Design review of the part built by this model. Coordinates are the model's own, in mm. Face numbers are marked on the shaded views. A direction names the side the tool comes from. Give positions to 0.01 mm unless a question says otherwise; leave off trailing zeros. Order: outer loops, then holes, each group sorted by start corner. A loop starts at its lowest first (then second) coordinate and runs counter-clockwise, first axis right, second up. Notation, with made-up numbers: (13.5, 58) -> (20.5, 58) arc R27 ccw to (20.5, 97) -> close; hole circle Ø7 at (39, 6.5). An arc over 180 degrees is marked (long way). Return JSON: item names as keys, results as strings.
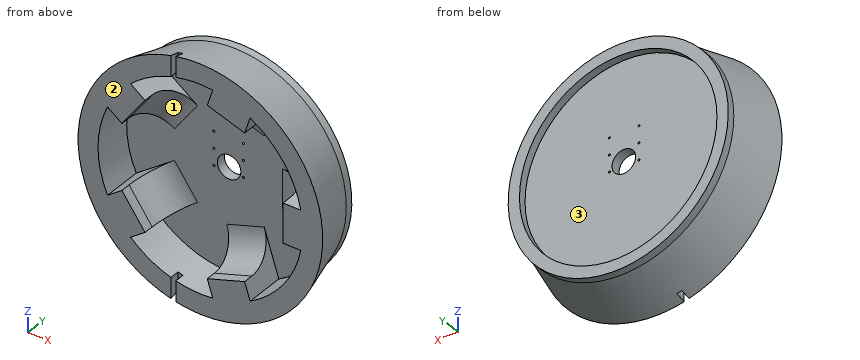
```python
from build123d import *

# Parameters (mm, degrees)
SKETCH10_R              = 1.025
CUT_EXTRUDE2_DEPTH      = 10
SKETCH11_R              = 112
SKETCH11_R_2            = 100.5
BOSS_EXTRUDE1_DEPTH     = 7.75
BOSS_EXTRUDE2_DEPTH     = 20
CIRPATTERN1_COUNT       = 5
CUT_EXTRUDE3_DEPTH      = 285.75526773
CUT_EXTRUDE3_DEPTH_BACK = 285.75526773
SKETCH14_W              = 5
SKETCH14_H              = 10


with BuildPart() as part:
    # Sketch4 → Revolve1 (revolve)
    with BuildSketch(Plane.XY, mode=Mode.PRIVATE) as revolve1_sk:
        Polygon((12, 50), (12, 40), (104.192235936, 40), (104.192235936, 0), (124.5, 0), (112, 50), align=None)
    revolve(revolve1_sk.sketch.rotate(Axis((0, 0, 0), (0, 1, 0)), 90), axis=Axis((0, 0, 0), (0, 1, 0)))

    # Sketch10 → Cut-Extrude2 (cut)
    with BuildSketch(Plane.XZ.offset(-40)):
        with Locations(Location((14.55, 12.4, 0), (0, 0, 270))):
            Circle(SKETCH10_R)
        with Locations(Location((-15.45, 12.4, 0), (0, 0, 270))):
            Circle(SKETCH10_R)
        with Locations(Location((-15.45, 29.4, 0), (0, 0, 270))):
            Circle(SKETCH10_R)
        with Locations(Location((14.55, 29.4, 0), (0, 0, 270))):
            Circle(SKETCH10_R)
        with Locations(Location((14.55, -4.6, 0), (0, 0, 270))):
            Circle(SKETCH10_R)
        with Locations(Location((-15.45, -4.6, 0), (0, 0, 270))):
            Circle(SKETCH10_R)
    extrude(amount=-CUT_EXTRUDE2_DEPTH, mode=Mode.SUBTRACT)

    # Sketch11 → Boss-Extrude1 (add)
    with BuildSketch(Plane(origin=(0, 50, 0), x_dir=(1, 0, 0), z_dir=(0, 1, 0))):
        with Locations(Location((0, 0, 0), (0, 0, 270))):
            Circle(SKETCH11_R)
        with Locations(Location((0, 0, 0), (0, 0, 270))):
            Circle(SKETCH11_R_2, mode=Mode.SUBTRACT)
    extrude(amount=BOSS_EXTRUDE1_DEPTH)

    # Sketch13 → Boss-Extrude2 (add, symmetric)
    with BuildSketch(Plane.XY):
        with BuildLine():
            ThreePointArc((84.192235936, 10), (75.405439372, 31.213203436), (54.192235936, 40))
            Line((54.192235936, 40), (104.192235936, 40))
            Line((104.192235936, 40), (104.192235936, 0))
            Line((104.192235936, 0), (84.192235936, 0))
            Line((84.192235936, 0), (84.192235936, 10))
        make_face()
    boss_extrude2 = extrude(amount=BOSS_EXTRUDE2_DEPTH, both=True)

    # CirPattern1: Boss-Extrude2 ×5 about axis
    cirpattern1_axis = Axis((0, 0, 0), (0, 1, 0))
    for i in range(1, CIRPATTERN1_COUNT):
        add(boss_extrude2.rotate(cirpattern1_axis, i * 360 / CIRPATTERN1_COUNT))

    # Sketch14 → Cut-Extrude3 (cut, two sides: drawn at the far end of the back side and taken through both)
    with BuildSketch(Plane.XY.offset(125).offset(-CUT_EXTRUDE3_DEPTH_BACK)):
        with Locations((-27.5, 5)):
            Rectangle(SKETCH14_W, SKETCH14_H)
    extrude(amount=CUT_EXTRUDE3_DEPTH + CUT_EXTRUDE3_DEPTH_BACK, mode=Mode.SUBTRACT)


solid = part.part
```
Item 1: Machinability: for the marked faces 1, 2 and 3, which of the approach directions +Z, -Z, +X, -X, +Y, -Y give a long, thin tool a straight path to every point of the face, cutting with its end or side? Answer none if there is none.
Result set:
{"face 1": "-Y", "face 2": "+Z, -Z, +X, -X, -Y", "face 3": "+Y"}
Item 2: Wall thickness on L1, parallel to X at y = 17, z = 35; L2, parallel to Y at x = -8, z = 91; L3, parallel to X at y = 44.25, z = 29.4 (3 decimals): over which ranges is each line inside the solid? List them lowest first. Write a range as [from, to].
Result set:
{"L1": "x = [-115.04, -98.14], [-82.2, -77.61], [98.14, 115.04]", "L2": "y = [40, 50]", "L3": "x = [-109.561, -16.475], [-14.425, 13.525], [15.575, 109.561]"}
Item 3: For pin 1 (3.5 mm diameter, centred on x = 14.55, z = 12.4, fed in from +Y); pin 2 (10 mm diameter, centred on x = -54.5, y = 8, fed in from +Z); pin 3 (1.8 mm diameter, centred on x = 14.55, z = 29.4, fed in from +Y); pin 4 (8 mm diameter, centred on y = 6.5, z = -9, fed in from -X), all flat-tipped, find the tip position at first contact; note any pin that passes through.
Result set:
{"pin 1": "stops at y = 50", "pin 2": "stops at z = 112.44", "pin 3": "passes through", "pin 4": "stops at x = -123.58"}
Item 4: Add section C-C (y = 29). Give the boundary of the cut face in (x, z).
Result set:
{"outline": "circle Ø234.5 at (0, 0); hole (-94.48, -43.92) -> (-74.38, -29.32) -> (-50.87, -61.68) -> (-70.97, -76.28) arc R104.19 ccw to (12.58, -103.43) -> (4.9, -79.8) -> (42.94, -67.44) -> (50.62, -91.07) arc R104.19 ccw to (102.25, -20) -> (77.41, -20) -> (77.41, 20) -> (102.25, 20) arc R104.19 ccw to (50.62, 91.07) -> (42.94, 67.44) -> (4.9, 79.8) -> (12.58, 103.43) arc R104.19 ccw to (-70.97, 76.28) -> (-50.87, 61.68) -> (-74.38, 29.32) -> (-94.48, 43.92) arc R104.19 ccw to start"}
Item 5: Add section A-A (z = 0). Give the boundary of the cut face in (x, y).
Result set:
{"outline": "(-124.5, 0) -> (-104.19, 0) -> (-104.19, 40) -> (-12, 40) -> (-12, 50) -> (-100.5, 50) -> (-100.5, 57.75) -> (-112, 57.75) -> (-112, 50) -> close; (12, 40) -> (54.19, 40) arc R30 cw to (84.19, 10) -> (84.19, 0) -> (124.5, 0) -> (112, 50) -> (112, 57.75) -> (100.5, 57.75) -> (100.5, 50) -> (12, 50) -> close"}
Item 6: Add section B-B (y = 16). Give the boundary of the cut face in (x, z), plus the area to 3 significant figures.
Result set:
{"outline": "circle Ø241 at (0, 0); hole (-94.48, -43.92) -> (-79.38, -32.95) -> (-55.87, -65.31) -> (-70.97, -76.28) arc R104.19 ccw to (12.58, -103.43) -> (6.81, -85.68) -> (44.85, -73.31) -> (50.62, -91.07) arc R104.19 ccw to (102.25, -20) -> (83.59, -20) -> (83.59, 20) -> (102.25, 20) arc R104.19 ccw to (50.62, 91.07) -> (44.85, 73.31) -> (6.81, 85.68) -> (12.58, 103.43) arc R104.19 ccw to (-70.97, 76.28) -> (-55.87, 65.31) -> (-79.38, 32.95) -> (-94.48, 43.92) arc R104.19 ccw to start", "area": "15,500 mm^2"}
